Can you work these out from the model? Positions are in its coordinate system, mm. Coordinates: 2 decimals unless noted, no trailing zeros. Order: outer loops, then holes, each group sorted by start corner. A loop starts at its lowest first (then second) coordinate and runs counter-clockwise, first axis right, second up. Notation, with made-up numbers: M -31.75,13.25 L 26.25,13.25 A20 cw 26.25,50.25 Z; hole C 83.5,26.5 d8. An arc over 180 degrees is marked long. Answer as CSV lines item,"result". Start each with the question number.
1. I need wall thicknesses on line 1 along Y through (x, z) = (0, 0.85); line 2 along Y through (x, z) = (9, 2.6); line 3 along Y through (x, z) = (10.75, 0.8). Which ranges of each line are inside material? Lowest first, please. Write a range as from..to.
2. If we section it at B-B (y = -9.25): List the corners of the cut face in (x, z) for me, plus the area to 3 significant figures.
3. If we section it at C-C (z = 1.6): List the corners of the cut face in (x, y) for me, plus the area to 3 significant figures.
4. If we section it at A-A (x = 0): List the corners of the cut face in (y, z) for me.
5. If we mould it in two halves opening along X, with no side actions, what happens to faces 1 (the face through (0, 12.5, 2)), 2 (the face through (-12.5, 0, 2)), 3 (the face through (10.387, -10.258, 1.622)), 4 (the face through (11, -11.07, 1.62))? For each: released by +X, released by -X, zero draft, split by the parting line, or undercut.
```python
from build123d import *

# Parameters (mm, degrees)
SKETCH1_W           = 25
SKETCH1_H           = 25
BOSS_EXTRUDE1_DEPTH = 3.2
CUT_EXTRUDE1_REACH  = 5.2
SKETCH2_R           = 6.32
SKETCH3_R           = 2.1
CUT_EXTRUDE2_DEPTH  = 4.2
CIRPATTERN1_COUNT   = 4
FILLET2_R           = 5


with BuildPart() as part:
    # Sketch1 → Boss-Extrude1 (new body)
    with BuildSketch(Plane.XY):
        Rectangle(SKETCH1_W, SKETCH1_H)
    extrude(amount=BOSS_EXTRUDE1_DEPTH)

    # Sketch2 → Cut-Extrude1 (cut, up to next)
    with BuildSketch(Plane.XY.offset(3.2), mode=Mode.PRIVATE) as cut_extrude1_sk1:
        Circle(SKETCH2_R)
    cut_extrude1_tool1 = extrude(cut_extrude1_sk1.sketch, amount=-CUT_EXTRUDE1_REACH, mode=Mode.PRIVATE) & part.part
    add(cut_extrude1_tool1.solids().sort_by_distance((0, 0, 3.2))[0], mode=Mode.SUBTRACT)

    # Sketch3 → Cut-Extrude2 (cut, through all)
    with BuildSketch(Plane.XY.offset(3.2)):
        with Locations((-8.838834765, 8.838834765)):
            Circle(SKETCH3_R)
    cut_extrude2 = extrude(amount=-CUT_EXTRUDE2_DEPTH, mode=Mode.SUBTRACT)

    # CirPattern1: Cut-Extrude2 ×4 about axis
    cirpattern1_axis = Axis((0, 0, 0), (0, 0, 1))
    for i in range(1, CIRPATTERN1_COUNT):
        add(cut_extrude2.rotate(cirpattern1_axis, i * 360 / CIRPATTERN1_COUNT), mode=Mode.SUBTRACT)

    # Fillet2
    fillet2_edges = [part.edges().sort_by_distance(p)[0] for p in [
        (12.5, -12.5, 1.6),
        (-12.5, -12.5, 1.6),
        (-12.5, 12.5, 1.6),
        (12.5, 12.5, 1.6),
    ]]
    fillet(fillet2_edges, radius=FILLET2_R)


solid = part.part
```
Solved:
1,line 1,"-12.5..-6.32, 6.32..12.5"
1,line 2,"-12.27..-10.93, -6.75..6.75, 10.93..12.27"
1,line 3,"-11.3..-9.71, -7.97..7.97, 9.71..11.3"
2,outline,"M -12.18,0 L -10.9,0 L -10.9,3.2 L -12.18,3.2 Z; M -6.78,0 L 6.78,0 L 6.78,3.2 L -6.78,3.2 Z; M 10.9,0 L 12.18,0 L 12.18,3.2 L 10.9,3.2 Z"
2,area,"51.6 mm²"
3,outline,"M -12.5,-7.5 A5 ccw -7.5,-12.5 L 7.5,-12.5 A5 ccw 12.5,-7.5 L 12.5,7.5 A5 ccw 7.5,12.5 L -7.5,12.5 A5 ccw -12.5,7.5 Z; hole C -8.84,-8.84 d4.2; hole C -8.84,8.84 d4.2; hole C 0,0 d12.64; hole C 8.84,-8.84 d4.2; hole C 8.84,8.84 d4.2"
3,area,"423 mm²"
4,outline,"M -12.5,0 L -6.32,0 L -6.32,3.2 L -12.5,3.2 Z; M 6.32,0 L 12.5,0 L 12.5,3.2 L 6.32,3.2 Z"
5,face 1,"zero draft"
5,face 2,"released by -X"
5,face 3,"undercut"
5,face 4,"released by +X"
